Part model, mm, in its own coordinate system. A direction names the side the tool comes from. Coordinates: 2 decimals unless noted, no trailing zeros. Write each loop counter-clockwise with the first axis right and the second up, starting at its lowest first coordinate (ties: lowest second). Pieces come first, ordered by that corner, then holes. Notation, with made-up numbers: M 6,54 L 53,54 A26 cw 53,73 Z; hole C 3,49 d6. An arc over 180 degrees is marked long. Use a Markdown table: item, result. Add a question column.
Q1. Mould opens along X. For faces 1 (the flat face through (-0.05, -0.5, -2.5)), 2 (the flat face through (0.72, 7.754, -2.046)), 3 (the flat face through (-1.32, 7.754, 2.046)), 4 (the flat face through (0.4, -0.5, 2)) say: released by +X, released by -X, zero draft, split by the parting line, or undercut.
Q2. Slice it at C-C on y = 5. Write the cut outline in (x, z).
Q3. Slice it at A-A on x = 2.45. Write the cut outline in (y, z).
Q4. Slice it at D-D on z = 0. Write the cut outline in (x, y), then the cut area to 3 significant figures.
Q5. Wall check: L1, parallel to Z at x = 2.25, y = 5.75; L2, parallel to Z at x = -0.3, y = 9; L3, parallel to X at y = 8.7, z = -2.5. Give the ranges that are in metal, low to high. Write a range as from..to.
Q6. Pin check, flat tips, straight feed: pin 1 Ø1.2 at (y, z) = (3.5, 3.5) entering from +X; pin 2 Ø0.5 at (y, z) = (-0.5, 2.5) entering from +X; pin 3 Ø0.8 at (x, y) = (0.5, -0.5) entering from +Z. Stop position of each tip, or through.
Q7. Slice it at B-B on x = -3.05. Write the cut outline in (y, z).
Q8. Tool access for faces 5 (the flat face through (0.4, -0.5, -2)), 6 (the flat face through (0.167, 7.754, 3.533)), 7 (the flat face through (3, 0.9, -2)), 8 (the flat face through (-0.05, -0.5, 2.5)): list every direction of +Z, -Z, +X, -X, +Y, -Y with a clear straight run to the whole face (end or side of a thin tool).
from build123d import *

# Parameters (mm, degrees)
BOSS_EXTRUDE1_DEPTH = 5
SKETCH2_W           = 1
SKETCH2_H           = 1
BOSS_EXTRUDE2_DEPTH = 1
SKETCH3_W           = 4
SKETCH3_H           = 5
CUT_EXTRUDE1_DEPTH  = 2
SKETCH4_R           = 1.75
SKETCH4_R_2         = 0.4
CUT_EXTRUDE2_DEPTH  = 2
CUT_EXTRUDE3_DEPTH  = 0.5
CHAMFER1_SIZE       = 0.3


with BuildPart() as part:
    # Sketch1 → Boss-Extrude1 (new body, symmetric)
    with BuildSketch(Plane.XY):
        Polygon((-3.75, 0), (3.75, 0), (3.75, 6.8), (1.75, 10), (-2.35, 10), (-3.75, 6.8), align=None)
    extrude(amount=BOSS_EXTRUDE1_DEPTH, both=True)

    # Sketch2 → Boss-Extrude2 (add)
    with BuildSketch(Plane.XZ):
        with Locations((0.45, 2.5)):
            Rectangle(SKETCH2_W, SKETCH2_H)
        with Locations((0.45, -2.5)):
            Rectangle(SKETCH2_W, SKETCH2_H)
    extrude(amount=BOSS_EXTRUDE2_DEPTH)

    # Sketch3 → Cut-Extrude1 (cut)
    with BuildSketch(Plane(origin=(3.75, 0, 0), x_dir=(0, 0, -1), z_dir=(1, 0, 0))):
        with Locations((-2.5, 3.4)):
            Rectangle(SKETCH3_W, SKETCH3_H)
        with Locations((2.5, 3.4)):
            Rectangle(SKETCH3_W, SKETCH3_H)
    extrude(amount=-CUT_EXTRUDE1_DEPTH, mode=Mode.SUBTRACT)

    # Sketch4 → Cut-Extrude2 (cut)
    with BuildSketch(Plane(origin=(0, 10, 0), x_dir=(1, 0, 0), z_dir=(0, 1, 0))):
        with Locations((-0.3, 2.5)):
            Circle(SKETCH4_R)
        with Locations((-0.3, -2.5)):
            Circle(SKETCH4_R)
        with Locations((2.45, 2.5)):
            Circle(SKETCH4_R_2)
        with Locations((2.45, -2.5)):
            Circle(SKETCH4_R_2)
        with Locations((-3.05, 2.5)):
            Circle(SKETCH4_R_2)
        with Locations((-3.05, -2.5)):
            Circle(SKETCH4_R_2)
    extrude(amount=-CUT_EXTRUDE2_DEPTH, mode=Mode.SUBTRACT)

    # Sketch5 → Cut-Extrude3 (cut)
    with BuildSketch(Plane(origin=(0, 8, 0), x_dir=(1, 0, 0), z_dir=(0, 1, 0))):
        with BuildLine():
            Line((-1.221836, -1.012479), (-0.3, -1.934315))
            Line((-0.3, -1.934315), (0.124264, -1.510051))
            Line((0.124264, -1.510051), (0.689949, -2.075736))
            Line((0.689949, -2.075736), (0.265685, -2.5))
            Line((0.265685, -2.5), (1.187521, -3.421836))
            ThreePointArc((1.187521, -3.421836), (0.937437, -3.737437), (0.621836, -3.987521))
            Line((0.621836, -3.987521), (-0.3, -3.065685))
            Line((-0.3, -3.065685), (-0.724264, -3.489949))
            Line((-0.724264, -3.489949), (-1.289949, -2.924264))
            Line((-1.289949, -2.924264), (-0.865685, -2.5))
            Line((-0.865685, -2.5), (-1.787521, -1.578164))
            ThreePointArc((-1.787521, -1.578164), (-1.537437, -1.262563), (-1.221836, -1.012479))
        make_face()
        with BuildLine():
            Line((-1.221836, 3.987521), (-0.3, 3.065685))
            Line((-0.3, 3.065685), (0.124264, 3.489949))
            Line((0.124264, 3.489949), (0.689949, 2.924264))
            Line((0.689949, 2.924264), (0.265685, 2.5))
            Line((0.265685, 2.5), (1.187521, 1.578164))
            ThreePointArc((1.187521, 1.578164), (0.937437, 1.262563), (0.621836, 1.012479))
            Line((0.621836, 1.012479), (-0.3, 1.934315))
            Line((-0.3, 1.934315), (-0.724264, 1.510051))
            Line((-0.724264, 1.510051), (-1.289949, 2.075736))
            Line((-1.289949, 2.075736), (-0.865685, 2.5))
            Line((-0.865685, 2.5), (-1.787521, 3.421836))
            ThreePointArc((-1.787521, 3.421836), (-1.537437, 3.737437), (-1.221836, 3.987521))
        make_face()
        with BuildLine():
            Line((-1.221836, -6.012479), (-0.3, -6.934315))
            Line((-0.3, -6.934315), (0.124264, -6.510051))
            Line((0.124264, -6.510051), (0.689949, -7.075736))
            Line((0.689949, -7.075736), (0.265685, -7.5))
            Line((0.265685, -7.5), (1.187521, -8.421836))
            ThreePointArc((1.187521, -8.421836), (0.937437, -8.737437), (0.621836, -8.987521))
            Line((0.621836, -8.987521), (-0.3, -8.065685))
            Line((-0.3, -8.065685), (-0.724264, -8.489949))
            Line((-0.724264, -8.489949), (-1.289949, -7.924264))
            Line((-1.289949, -7.924264), (-0.865685, -7.5))
            Line((-0.865685, -7.5), (-1.787521, -6.578164))
            ThreePointArc((-1.787521, -6.578164), (-1.537437, -6.262563), (-1.221836, -6.012479))
        make_face()
    extrude(amount=-CUT_EXTRUDE3_DEPTH, mode=Mode.SUBTRACT)

    # Chamfer1
    chamfer1_edges = [part.edges().sort_by_distance(p)[0] for p in [
        (3.75, 3.4, 4.5),
        (3.75, 0.9, 2.5),
        (3.75, 3.4, 0.5),
        (3.75, 5.9, 2.5),
        (3.75, 3.4, -0.5),
        (3.75, 0.9, -2.5),
        (3.75, 3.4, -4.5),
        (3.75, 5.9, -2.5),
    ]]
    chamfer(chamfer1_edges, length=CHAMFER1_SIZE)


solid = part.part
Recorded:
| question | item | result |
|---|---|---|
| 1 | face 1 | released by -X |
| 1 | face 2 | undercut |
| 1 | face 3 | undercut |
| 1 | face 4 | zero draft |
| 2 | outline | M -3.75,-5 L 3.75,-5 L 3.75,-4.8 L 3.45,-4.5 L 1.75,-4.5 L 1.75,-0.5 L 3.45,-0.5 L 3.75,-0.2 L 3.75,0.2 L 3.45,0.5 L 1.75,0.5 L 1.75,4.5 L 3.45,4.5 L 3.75,4.8 L 3.75,5 L -3.75,5 Z |
| 3 | outline | M 0,-5 L 8.88,-5 L 8.88,-2.9 L 8,-2.9 L 8,-2.1 L 8.88,-2.1 L 8.88,2.1 L 8,2.1 L 8,2.9 L 8.88,2.9 L 8.88,5 L 0,5 Z; hole M 0.9,-4.5 L 5.9,-4.5 L 5.9,-0.5 L 0.9,-0.5 Z; hole M 0.9,0.5 L 5.9,0.5 L 5.9,4.5 L 0.9,4.5 Z |
| 4 | outline | M -3.75,0 L 3.75,0 L 3.75,6.8 L 1.75,10 L -2.35,10 L -3.75,6.8 Z |
| 4 | area | 69.6 mm² |
| 5 | L1 | -5..-4.5, -0.5..0.5, 4.5..5 |
| 5 | L2 | -5..-4.25, -0.75..0.75, 4.25..5 |
| 5 | L3 | -2.65..-2.05, 1.45..2.05 |
| 6 | pin 1 | x = 1.75 |
| 6 | pin 2 | x = 0.95 |
| 6 | pin 3 | z = 3 |
| 7 | outline | M 0,-5 L 8.4,-5 L 8.4,-2.9 L 8,-2.9 L 8,-2.1 L 8.4,-2.1 L 8.4,2.1 L 8,2.1 L 8,2.9 L 8.4,2.9 L 8.4,5 L 0,5 Z |
| 8 | face 5 | +X, -X, -Y |
| 8 | face 6 | +Y |
| 8 | face 7 | +X |
| 8 | face 8 | +Z, -Z, -X, -Y |
